from build123d import *

# Parameters (mm, degrees)
BOSS_EXTRUDE1_DEPTH = 10
SKETCH3_W           = 45
SKETCH3_H           = 21
BOSS_EXTRUDE2_DEPTH = 2
SKETCH4_R           = 1.5
CUT_EXTRUDE1_DEPTH  = 5


with BuildPart() as part:
    # Sketch2 → Boss-Extrude1 (new body)
    with BuildSketch(Plane.XY):
        Polygon((-17.5, 0), (-17.5, -1), (-14.5, -1), (-14.5, -5), (-22.5, -5), (-22.5, 0), (-22.5, 4), (22.5, 4), (22.5, -5), (14.5, -5), (14.5, -1), (17.5, -1), (17.5, 0), align=None)
    extrude(amount=BOSS_EXTRUDE1_DEPTH)

    # Sketch3 → Boss-Extrude2 (add)
    with BuildSketch(Plane(origin=(0, 4, 0), x_dir=(1, 0, 0), z_dir=(0, 1, 0))):
        with Locations((0, -5)):
            Rectangle(SKETCH3_W, SKETCH3_H)
    extrude(amount=BOSS_EXTRUDE2_DEPTH)

    # Sketch4 → Cut-Extrude1 (cut)
    with BuildSketch(Plane(origin=(0, 6, 0), x_dir=(1, 0, 0), z_dir=(0, 1, 0))):
        with Locations((-15.5, -13)):
            Circle(SKETCH4_R)
        with Locations((-15.5, 3)):
            Circle(SKETCH4_R)
        with Locations((15.5, 3)):
            Circle(SKETCH4_R)
        with Locations((15.5, -13)):
            Circle(SKETCH4_R)
    extrude(amount=-CUT_EXTRUDE1_DEPTH, mode=Mode.SUBTRACT)


solid = part.part
Design review of the part built by this model. Coordinates are the model's own, in mm. A direction names the side the tool comes from. Give positions to 0.01 mm unless a question says otherwise; leave off trailing zeros. Write each loop counter-clockwise with the first axis right and the second up, starting at its lowest first coordinate (ties: lowest second). Pieces come first, ordered by that corner, then holes. Notation, with made-up numbers: M -31,16 L -6,16 A15 ccw -6,39 Z; hole C 53,-18.5 d10. An arc over 180 degrees is marked long. Answer as a JSON object with one key per item and string values. Group by question number.
1) We need section A-A (x = -15.5). Give the boundary of the cut face in (y, z).
2) We need section B-B (y = -3.5). Give the boundary of the cut face in (x, z), and give its area (3 significant figures).
3) We need section C-C (z = -3). Give the boundary of the cut face in (x, y).
4) Mouldability with a two-part tool opening along Z and no side actions: class faces 1 (the face through (14, 5, 13)), 2 (the face through (0, 1, 10)), 3 (the face through (-22.5, 2, 5)) as released by +Z, released by -Z, zero draft, split by the parting line, or undercut.
5) Tool access review of faces 4 (the face through (0, 1, 0)), 5 (the face through (-14.5, -3, 5)), 6 (the face through (0, 4, 13)), 7 (the face through (0, 0, 5)), 8 (the face through (-18, -5, 5)): name each direction out of +Z, -Z, +X, -X, +Y, -Y from which nothing blocks a thin tool from reaching the whole face with its end or side.
6) Clearance check with flat-ended pins moving along their axes: pin 1 Ø4.5 at (x, y) = (-10.5, 0) entering from -Z; pin 2 Ø5 at (x, z) = (15.5, -3) entering from -Y; pin 3 Ø4.5 at (x, z) = (-3, 11.5) entering from -Y. State where each tip first meets the part, or that it passes through.
7) We need section D-D (y = 5.25). Give the boundary of the cut face in (x, z), and give its area (3 significant figures).
8) For line 1 along Z through (x, y) = (15.5, 4.6); line 2 along X through (y, z) = (5.45, -3); line 3 along Y through (x, z) = (17, 3.25), list the stretches that pass through material, from the lowest coordinate up.
Answer key:
{
 "1": {"outline": "M -5,0 L -1,0 L -1,10 L -5,10 Z; M 0,0 L 4,0 L 4,-1.5 L 6,-1.5 L 6,11.5 L 4,11.5 L 4,10 L 0,10 Z; M 4,-5.5 L 6,-5.5 L 6,-4.5 L 4,-4.5 Z; M 4,14.5 L 6,14.5 L 6,15.5 L 4,15.5 Z"},
 "2": {"outline": "M -22.5,0 L -14.5,0 L -14.5,10 L -22.5,10 Z; M 14.5,0 L 22.5,0 L 22.5,10 L 14.5,10 Z", "area": "160 mm²"},
 "3": {"outline": "M -22.5,4 L -17,4 L -17,6 L -22.5,6 Z; M -14,4 L 14,4 L 14,6 L -14,6 Z; M 17,4 L 22.5,4 L 22.5,6 L 17,6 Z"},
 "4": {"face 1": "undercut", "face 2": "released by +Z", "face 3": "zero draft"},
 "5": {"face 4": "-Z, +X, -X, -Y", "face 5": "+Z, -Z, -Y", "face 6": "+Z, +X, -X, -Y", "face 7": "+Z, -Z", "face 8": "+Z, -Z, +X, -X, -Y"},
 "6": {"pin 1": "stops at z = 0", "pin 2": "stops at y = 4", "pin 3": "stops at y = 0"},
 "7": {"outline": "M -22.5,-5.5 L 22.5,-5.5 L 22.5,15.5 L -22.5,15.5 Z; hole C -15.5,-3 d3; hole C -15.5,13 d3; hole C 15.5,-3 d3; hole C 15.5,13 d3", "area": "917 mm²"},
 "8": {"line 1": "z = -5.5 to -4.5, -1.5 to 11.5, 14.5 to 15.5", "line 2": "x = -22.5 to -17, -14 to 14, 17 to 22.5", "line 3": "y = -5 to -1, 0 to 6"}
}
